The drawing under review shows one solid part. Ordinate dimensions are in mm from its lowest x, y, z. Give positions to 0.01 mm unless a question says otherwise; leave off trailing zeros. Write each loop counter-clockwise with the first axis right and the second up, starting at its lowest first coordinate (ties: lowest second). Pieces come first, ordered by that corner, then holes.
Q1. Insertion check: P1, Ø2, axis at x = 24.5, y = 15.5, coming from the -Z side. The pin has a flat end and moves straight along its axis. Give the tip position at first contact, or say it passes through.
Q2. We need section B-B (x = 14.4). Write out the cut boundary in (y, z).
Q3. We need section C-C (z = 6.5). Write out the cut boundary in (x, y), then the cut area to 3 significant figures.
Q4. Mouldability with a two-part tool opening along Y and no side actions: class the marked faces 1, 2 and 3 as released by +Y, released by -Y, zero draft, split by the parting line, or undercut.
Q5. For line 1 (Y direction, x = 14.4, z = 3.25); line 2 (X direction, y = 15.5, z = 6); line 3 (Y direction, x = 16, z = 1.75), list the stretches that pass through material, from the lowest coordinate up.
Q6. We need section A-A (y = 15.34). Write out the cut boundary in (x, z), then the cut area to 3 significant figures.
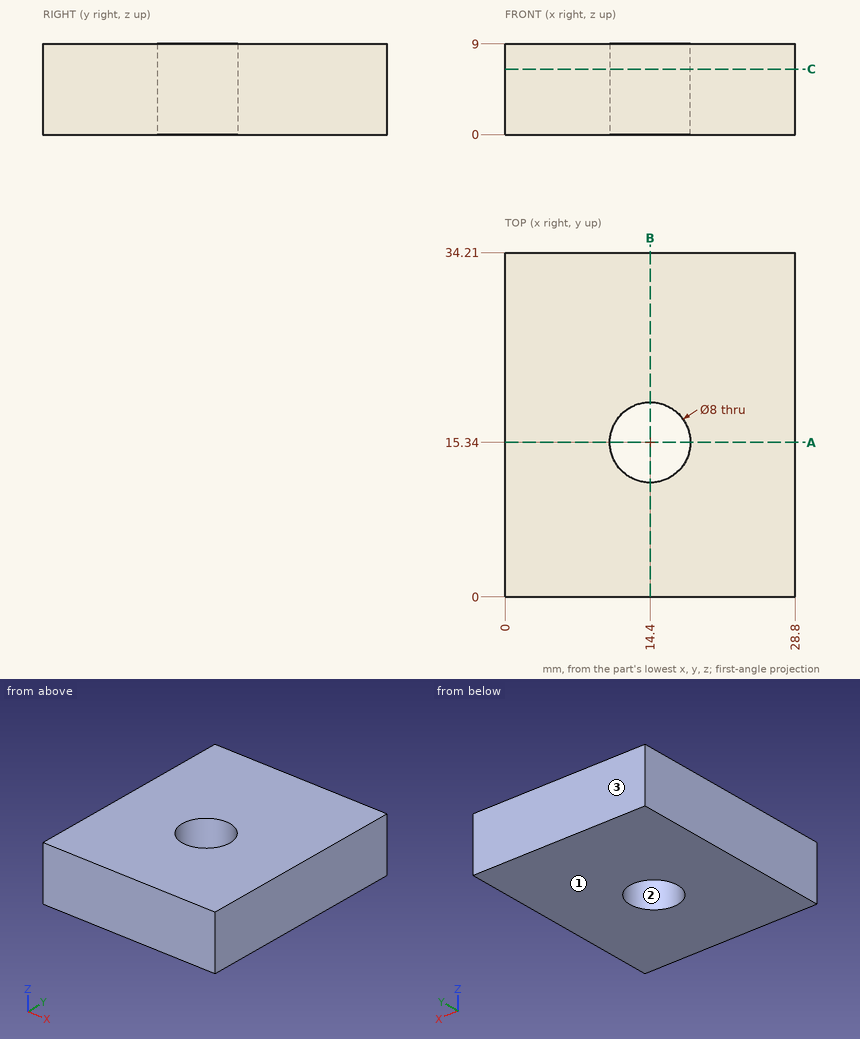
Computed:
1. P1: stops at z = 0
2. outline: (0, 0) - (11.34, 0) - (11.34, 9) - (0, 9) - close; (19.34, 0) - (34.21, 0) - (34.21, 9) - (19.34, 9) - close
3. outline: (0, 0) - (28.8, 0) - (28.8, 34.21) - (0, 34.21) - close; hole circle Ø8 at (14.4, 15.34)
3. area: 935 mm2
4. face 1: zero draft
4. face 2: undercut
4. face 3: released by +Y
5. line 1: y = 0 to 11.34, 19.34 to 34.21
5. line 2: x = 0 to 10.4, 18.4 to 28.8
5. line 3: y = 0 to 11.67, 19.01 to 34.21
6. outline: (0, 0) - (10.4, 0) - (10.4, 9) - (0, 9) - close; (18.4, 0) - (28.8, 0) - (28.8, 9) - (18.4, 9) - close
6. area: 187 mm2
